CAD build for the part. Positions are in the model's coordinates, mm. Round coordinates to 2 decimals unless told otherwise and drop trailing zeros. Order: outer loops, then holes, each group sorted by start corner. A loop starts at its lowest first (then second) coordinate and runs counter-clockwise, first axis right, second up. Notation, with made-up numbers: M 12.25,3.25 L 17.25,3.25 A14 ccw 17.25,23.25 Z; hole C 16,-29.75 d5. An arc over 180 degrees is marked long. Put each result on its own line as item: value.
```python
from build123d import *

# Parameters (mm, degrees)
F1_DEPTH = 24
F2_R     = 2.5
F3_DEPTH = 25


with BuildPart() as f1:
    # F0 (on Top) → F1 (new body)
    with BuildSketch(Plane.XY):
        with BuildLine():
            Line((16.125, 0), (19, 0))
            ThreePointArc((19, 0), (0, 19), (-19, 0))
            Line((-19, 0), (-16.125, 0))
            ThreePointArc((-16.125, 0), (0, 16.125), (16.125, 0))
        make_face()
    extrude(amount=F1_DEPTH)

    # F2 (on Front) → F3 (cut)
    with BuildSketch(Plane.XZ):
        with Locations((0, 12)):
            Circle(F2_R)
    extrude(amount=-F3_DEPTH, mode=Mode.SUBTRACT)


solid = f1.part
```
Item 1: Pin check, flat tips, straight feed: P1, Ø1.5, axis at y = 15.5, z = 13.5, coming from the -X side; P2, Ø1, axis at y = 5, z = 13, coming from the -X side; P3, Ø6, axis at y = 12, z = 5.5, coming from the -X side. Stop position of each tip, or through.
Answers below:
P1: x = -11.98
P2: x = -18.46
P3: x = -16.73
Item 2: Band-saw the part on A-A on x = 0. Give the cut face in (y, z) (3 decimals).
Answers below:
outline: M 16.125,0 L 19,0 L 19,9.5 L 16.125,9.5 Z; M 16.125,14.5 L 19,14.5 L 19,24 L 16.125,24 Z
Item 3: Probe line 1 along Z through (x, y) = (0, 17.7); line 2 along X through (y, z) = (7, 17.25); line 3 along Y through (x, z) = (0, 4.25) (3 decimals). List the from-to ranges inside material, lowest first. Write a range as [from, to].
Answers below:
line 1: [0, 9.5], [14.5, 24]
line 2: [-17.66, -14.53], [14.53, 17.66]
line 3: [16.125, 19]
Item 4: Band-saw the part on D-D on x = 14. Give the cut face in (y, z).
Answers below:
outline: M 8,0 L 12.85,0 L 12.85,24 L 8,24 Z
Item 5: Mould opens along X. For faces 1 (the cylindrical face through (0, 19, 9)), 2 (the flat face through (-18, 0, 12)), 3 (the cylindrical face through (-0.35, 16.12, 9.17)), 4 (the cylindrical face through (-0.33, 17.44, 14.48)) say: pulls with the +X half, pulls with the -X half, needs draft (parallel to the pull), parting line crosses it, or undercut.
Answers below:
face 1: parting line crosses it
face 2: needs draft
face 3: undercut
face 4: undercut
Item 6: Band-saw the part on B-B on y = 9.25. Give the cut face in (x, z).
Answers below:
outline: M -16.6,0 L -13.21,0 L -13.21,24 L -16.6,24 Z; M 13.21,0 L 16.6,0 L 16.6,24 L 13.21,24 Z
Item 7: Band-saw the part on C-C on z = 21. Give the cut face in (x, y) (3 decimals).
Answers below:
outline: M -19,0 L -16.125,0 A16.125 cw 16.125,0 L 19,0 A19 ccw Z
